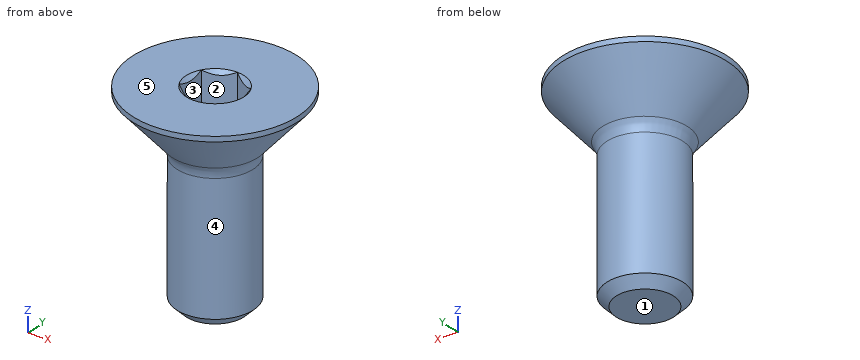
```python
from build123d import *

# Parameters (mm, degrees)
SKETCH1_W          = 12.7
SKETCH1_H          = 2.413
CHAMFER1_SIZE      = 0.5953125
CUT_EXTRUDE2_DEPTH = 2.25806


with BuildPart() as part:
    # Sketch1 → Revolve1 (revolve)
    with BuildSketch(Plane(origin=(0, 0, 0), x_dir=(0, 0, -1), z_dir=(1, 0, 0))):
        with Locations((6.35, 1.2065)):
            Rectangle(SKETCH1_W, SKETCH1_H)
    revolve(axis=Axis((0, 0, -12.7), (0, 0, 1)))

    # Chamfer1
    chamfer1_edges = [part.edges().sort_by_distance(p)[0] for p in [
        (0, -2.413, -12.7),
    ]]
    chamfer(chamfer1_edges, length=CHAMFER1_SIZE)


with BuildPart() as body_2:
    # Sketch7 → Revolve2 (revolve)
    with BuildSketch(Plane(origin=(0, 0, 0), x_dir=(0, 0, -1), z_dir=(1, 0, 0)), mode=Mode.PRIVATE) as revolve2_sk:
        with BuildLine():
            Line((0, 5.2197), (0.32258, 5.2197))
            Line((0.32258, 5.2197), (3.2258, 2.695969357))
            ThreePointArc((3.2258, 2.695969357), (3.578633365, 2.486055564), (3.982635924, 2.413))
            Line((3.982635924, 2.413), (3.982635924, 0))
            Line((3.982635924, 0), (0, 0))
            Line((0, 0), (0, 5.2197))
        make_face()
    revolve(revolve2_sk.sketch.rotate(Axis((0, 0, 0), (0, 0, -1)), 180), axis=Axis((0, 0, 0), (0, 0, -1)))

    # Boss-Extrude1 cone 1 section (through the dimple's axis) → Boss-Extrude1 (revolve)
    with BuildSketch(Plane(origin=(0, 0, -3.982635924), x_dir=(0, -1, 0), z_dir=(1, 0, 0))):
        Polygon((0, 0), (2.413, 0), (0, 2.413), align=None)
    revolve(axis=Axis((0, 0, -3.982635924), (0, 0, -1)))

    # Combine1: union part
    add(part.part)

    # Sketch5 → Cut-Extrude2 (cut)
    with BuildSketch(Plane.XY):
        Polygon((1.5875, -0.916543552), (1.5875, 0.916543552), (0, 1.833087105), (-1.5875, 0.916543552), (-1.5875, -0.916543552), (0, -1.833087105), align=None)
    extrude(amount=-CUT_EXTRUDE2_DEPTH, mode=Mode.SUBTRACT)

    # Cut-Extrude3 cone 1 section (through the dimple's axis) → Cut-Extrude3 (revolve, cut)
    with BuildSketch(Plane(origin=(0, 0, 0), x_dir=(0, -1, 0), z_dir=(1, 0, 0))):
        Polygon((0, 0), (1.833087105, 0), (0, 1.833087105), align=None)
    revolve(axis=Axis((0, 0, 0), (0, 0, -1)), mode=Mode.SUBTRACT)


solid = body_2.part
```
Could you check a few things on this model? Use its own coordinates, in mm. Face numbers are marked on the shaded views. A direction names the side the tool comes from. Give positions to 0.01 mm unless a question says otherwise; leave off trailing zeros. Order: outer loops, then holes, each group sorted by start corner. A loop starts at its lowest first (then second) coordinate and runs counter-clockwise, first axis right, second up.
Q1. Suppose I cut it at A-A, the plane y = 0. Write out the boundary of the cut face in (x, z), and give its area (3 significant figures).
Q2. Suppose I cut it at B-B, the plane z = -6.25. Write out the boundary of the cut face in (x, y), and give its area (3 significant figures).
Q3. If I drill on line 1 along Y through (x, z) = (-3.75, -0.75); line 2 along Y through (x, z) = (2, -7.75); line 3 along Z through (x, y) = (-3, -1.75), over which ranges is the centre line in solid material (lowest first)?
Q4. We'd pull the mould along X, two halves only. Please class the marked faces 3, 4 and 5: +X half, -X half, draft (parallel to the pull), parting line (faces both ways), or undercut.
Q5. For the marked faces 1 and 2, which set-ups out of +Z, -Z, +X, -X, +Y, -Y let a thin tool reach every point of the face, with its end or its side?
Q6. I'm going to push flat-ended pins straight in: P1, Ø0.5, axis at y = -0.5, z = -1.5, coming from the -X side; P2, Ø5, axis at x = -2.5, z = -11, coming from the -Y side; P3, Ø1, axis at x = -2, y = -1.5, coming from the -Z side. Where does each tip first touch, or does it pass through?
Solution:
1. outline: (-5.22, -0.32) - (-2.7, -3.23) arc R1.15 cw to (-2.41, -3.98) - (-2.41, -12.1) - (-1.82, -12.7) - (1.82, -12.7) - (2.41, -12.1) - (2.41, -3.98) arc R1.15 cw to (2.7, -3.23) - (5.22, -0.32) - (5.22, 0) - (1.83, 0) - (1.59, -0.25) - (1.59, -2.26) - (-1.59, -2.26) - (-1.59, -0.25) - (-1.83, 0) - (-5.22, 0) - close
1. area: 64.6 mm2
2. outline: circle Ø4.83 at (0, 0)
2. area: 18.3 mm2
3. line 1: y = -3.07 to 3.07
3. line 2: y = -1.35 to 1.35
3. line 3: z = -2.33 to 0
4. face 3: undercut
4. face 4: parting line
4. face 5: draft
5. face 1: -Z, +X, -X, +Y, -Y
5. face 2: +Z
6. P1: stops at x = -4.39
6. P2: stops at y = -2.41
6. P3: stops at z = -12.52
